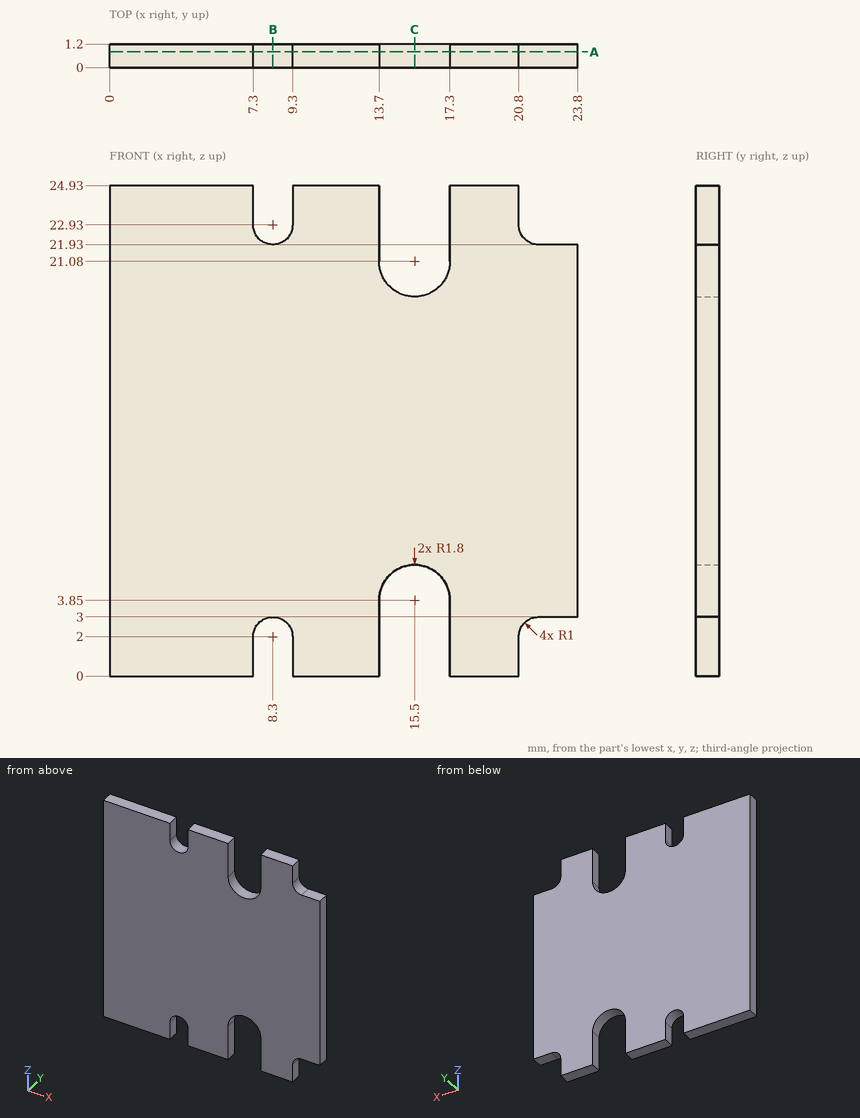
Input: dimensioned drawing with shaded views. Units: mm. Origin: part minimum x, y, z. Coordinates: 2 decimals unless noted, no trailing zeros. Order: outer loops, then holes, each group sorted by start corner. A loop starts at its lowest first (then second) coordinate and runs counter-clockwise, first axis right, second up. Notation, with made-up numbers: M 1,-5 L 5,-5 A31 ccw 5,22 Z; hole C -27.75,67.5 d1. An arc over 180 degrees is marked long. Write each question's results on one line, items separated by ' | '. Start each with the question number.
Item 1: Cut plane A-A (y = 0.8). Return loops of the section in (x, z), and give its area (3 significant figures).
Item 2: Cut plane C-C (x = 15.5). Return loops of the section in (y, z), and give its area (3 significant figures).
Item 3: First-contact query: pin 1 Ø0.6 at (y, z) = (0.5, 1) entering from -X. Flat tip, straight axial feed; report the tip coordinate or a pass-through.
Item 4: Cut plane B-B (x = 8.3). Return loops of the section in (y, z).
Item 5: Line query: probe 1 along X at (y, z) = (1.1, 1.5); probe 2 along X at (y, z) = (1.15, 21); probe 3 along Z at (x, y) = (22, 0.25). Output: solid intervals per line, ascending.
Checked values:
1) outline: M 0,0 L 7.3,0 L 7.3,2 A1 cw 9.3,2 L 9.3,0 L 13.7,0 L 13.7,3.85 A1.8 cw 17.3,3.85 L 17.3,0 L 20.8,0 L 20.8,2 A1 cw 21.8,3 L 23.8,3 L 23.8,21.93 L 21.8,21.93 A1 cw 20.8,22.93 L 20.8,24.93 L 17.3,24.93 L 17.3,21.08 A1.8 cw 13.7,21.08 L 13.7,24.93 L 9.3,24.93 L 9.3,22.93 A1 cw 7.3,22.93 L 7.3,24.93 L 0,24.93 Z | area: 527 mm2
2) outline: M 0,5.65 L 1.2,5.65 L 1.2,19.28 L 0,19.28 Z | area: 16.4 mm2
3) pin 1: stops at x = 0
4) outline: M 0,3 L 1.2,3 L 1.2,21.93 L 0,21.93 Z
5) probe 1: x = 0 to 7.3, 9.3 to 13.7, 17.3 to 20.8 | probe 2: x = 0 to 13.7, 17.3 to 23.8 | probe 3: z = 3 to 21.93
